Read the model definition and answer for the solid it produces. Units are mm, in the model's axes. A direction names the side the tool comes from. Round coordinates to 2 decimals unless told otherwise and drop trailing zeros. Order: outer loops, then holes, each group sorted by start corner. A loop starts at its lowest first (then second) coordinate and runs counter-clockwise, first axis right, second up. Notation, with made-up numbers: (58.5, 10.5) - (86.5, 10.5) arc R5 cw to (86.5, 19.5) - close; hole circle Ø7 at (86, 58). An arc over 180 degrees is marked (long way). One line per question, with ' | ' between items. Start each with the question number.
1) The part is cut by section B-B, the plane y = 27.5. Give the vertices of the cut face in (x, z).
2) The mould has two halves that part along X. Classify faces 1 (the flat face through (-95.25, 45, 17)), 2 (the flat face through (95.25, 45, 17)), 3 (the flat face through (-1, 78, 5.08)): pulls with the +X half, pulls with the -X half, needs draft (parallel to the pull), parting line crosses it, or undercut.
3) The part is cut by section A-A, the plane z = 30.5. Give the vertices of the cut face in (x, y).
4) The part is cut by section C-C, the plane x = -68.5. Give the vertices of the cut face in (y, z).
5) For faces 4 (the flat face through (-1, 46, 0)), 5 (the flat face through (-1, 34, 5.08)), determine the directions among +Z, -Z, +X, -X, +Y, -Y from which every point of the face is accessible in a straight line to the end or side of a thin tool.
6) Straight lines are drawn through the part: line 1 (Y direction, x = 50.5, z = 18); line 2 (X direction, y = 78, z = 12); line 3 (Z direction, x = -14, y = 68). For each, find the intervals that lie inside material, in ascending order. Write a range as from..to.
from build123d import *

# Parameters (mm, degrees)
F0_W     = 190.5
F0_H     = 101.6
F0_W_2   = 175.26
F0_H_2   = 2.54
F1_DEPTH = 33.02
F0_H_3   = 31.75
F0_H_4   = 52.07
F2_DEPTH = 5.08
F3_W     = 190.5
F3_H     = 10.465697
F4_DEPTH = 33.02


with BuildPart() as f1:
    # F0 (on Top) → F1 (new body)
    with BuildSketch(Plane.XY):
        with Locations((0, 50.8)):
            Rectangle(F0_W, F0_H)
        Polygon((87.63, 7.62), (-87.63, 7.62), (-87.63, 59.69), (-87.63, 62.23), (-87.63, 93.98), (87.63, 93.98), (87.63, 62.23), (87.63, 59.69), align=None, mode=Mode.SUBTRACT)
        with Locations((0, 60.96)):
            Rectangle(F0_W_2, F0_H_2)
    extrude(amount=F1_DEPTH)

    # F0 (on Top) → F2 (join)
    with BuildSketch(Plane.XY):
        with Locations((0, 78.105)):
            Rectangle(F0_W_2, F0_H_3)
        with Locations((0, 33.655)):
            Rectangle(F0_W_2, F0_H_4)
    extrude(amount=F2_DEPTH)

    # F3 (on face) → F4 (join)
    with BuildSketch(Plane.XY.offset(33.02)):
        with Locations((0, -5.232848)):
            Rectangle(F3_W, F3_H)
    extrude(amount=-F4_DEPTH)


solid = f1.part
Values:
1) outline: (-95.25, 0) - (95.25, 0) - (95.25, 33.02) - (87.63, 33.02) - (87.63, 5.08) - (-87.63, 5.08) - (-87.63, 33.02) - (-95.25, 33.02) - close
2) face 1: pulls with the -X half | face 2: pulls with the +X half | face 3: undercut
3) outline: (-95.25, -10.47) - (95.25, -10.47) - (95.25, 101.6) - (-95.25, 101.6) - close; hole (-87.63, 7.62) - (87.63, 7.62) - (87.63, 59.69) - (-87.63, 59.69) - close; hole (-87.63, 62.23) - (87.63, 62.23) - (87.63, 93.98) - (-87.63, 93.98) - close
4) outline: (-10.47, 0) - (101.6, 0) - (101.6, 33.02) - (93.98, 33.02) - (93.98, 5.08) - (62.23, 5.08) - (62.23, 33.02) - (59.69, 33.02) - (59.69, 5.08) - (7.62, 5.08) - (7.62, 33.02) - (-10.47, 33.02) - close
5) face 4: -Z, +X, -X, +Y, -Y | face 5: +Z
6) line 1: y = -10.47..7.62, 59.69..62.23, 93.98..101.6 | line 2: x = -95.25..-87.63, 87.63..95.25 | line 3: z = 0..5.08
